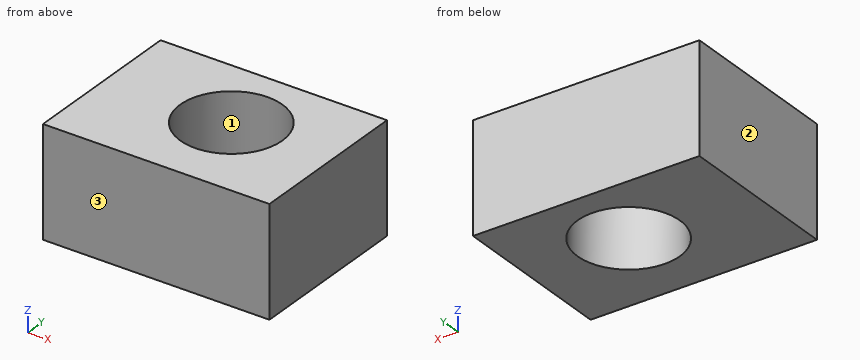
```python
from build123d import *

# Parameters (mm, degrees)
F0_W     = 15.52
F0_H     = 11.443967
F0_R     = 3.5
F1_DEPTH = 3.75


with BuildPart() as f1:
    # F0 (on Top) → F1 (new body, symmetric)
    with BuildSketch(Plane.XY):
        with Locations((-35.109139, 23.954742)):
            Rectangle(F0_W, F0_H)
        with Locations((-34.331899, 24.439655)):
            Circle(F0_R, mode=Mode.SUBTRACT)
    extrude(amount=F1_DEPTH, both=True)


solid = f1.part
```
Geometry check sheet. Reference: the model listing, model coordinates, mm. Face numbers are marked on the shaded views. Give positions to 0.01 mm unless a question says otherwise; leave off trailing zeros. Loops run counter-clockwise (first coordinate to the right, second up) from the corner with the lowest first, then second, coordinate; pieces in that order, holes last. Notation, with made-up numbers: M 49.25,82 L 86.25,82 A14 cw 86.25,108 Z; hole C 19.5,-5 d2. An arc over 180 degrees is marked long. Write item = value, one per line. Start each with the question number.
1. Thickness scan on probe 1 along Y at (x, z) = (-34.5, 2.75); probe 2 along Y at (x, z) = (-36.5, -2.25); probe 3 along X at (y, z) = (23.75, -1). Record the ranges inside material, lowest first.
2. Draft check along Y on the marked faces 1, 2 and 3. Enter one of: +Y half, -Y half, draft (parallel to the pull), parting line (faces both ways), or undercut.
3. Section check B-B, the plane y = 27.75. Enter the section's corners in (x, z).
4. Section check A-A, the plane x = -36. Enter the section's corners in (y, z).
5. Section check C-C, the plane z = -0.5. Enter the section's corners in (x, y), plus the area to 3 significant figures.
Values follow:
q1.probe_1 = 18.23 to 20.94, 27.94 to 29.68
q1.probe_2 = 18.23 to 21.69, 27.19 to 29.68
q1.probe_3 = -42.87 to -37.76, -30.9 to -27.35
q2.face_1 = undercut
q2.face_2 = draft
q2.face_3 = -Y half
q3.outline = M -42.87,-3.75 L -35.47,-3.75 L -35.47,3.75 L -42.87,3.75 Z; M -33.2,-3.75 L -27.35,-3.75 L -27.35,3.75 L -33.2,3.75 Z
q4.outline = M 18.23,-3.75 L 21.36,-3.75 L 21.36,3.75 L 18.23,3.75 Z; M 27.52,-3.75 L 29.68,-3.75 L 29.68,3.75 L 27.52,3.75 Z
q5.outline = M -42.87,18.23 L -27.35,18.23 L -27.35,29.68 L -42.87,29.68 Z; hole C -34.33,24.44 d7
q5.area = 139 mm^2
